```python
from build123d import *

# Parameters (mm, degrees)
SKETCH1_W           = 82.55
SKETCH1_H           = 69.85
BOSS_EXTRUDE1_DEPTH = 19.05
CUT_EXTRUDE2_START  = -19.05
SKETCH2_R           = 5.159375
CUT_EXTRUDE2_DEPTH  = 77.376117521
CUT_EXTRUDE4_START  = -19.05
SKETCH3_R           = 7.3421875
CUT_EXTRUDE4_DEPTH  = 28.575
CUT_EXTRUDE6_START  = -19.05
SKETCH4_R           = 12.7254
CUT_EXTRUDE6_DEPTH  = 2.8194
CUT_EXTRUDE8_START  = 41.275
SKETCH5_R           = 7.3421875
CUT_EXTRUDE8_DEPTH  = 60.325


with BuildPart() as part:
    # Sketch1 → Boss-Extrude1 (new, symmetric)
    with BuildSketch(Plane(origin=(0, 0, 0), x_dir=(1, 0, 0), z_dir=(0, 1, 0))):
        Rectangle(SKETCH1_W, SKETCH1_H)
    extrude(amount=BOSS_EXTRUDE1_DEPTH, both=True)

    # Sketch2 → Cut-Extrude2 (cut, through all)
    with BuildSketch(Plane(origin=(0, 0, 0), x_dir=(1, 0, 0), z_dir=(0, 1, 0)).offset(CUT_EXTRUDE2_START)):
        with Locations(Location((-30.1625, -23.8125, 0), (0, 0, 270))):
            Circle(SKETCH2_R)
        with Locations(Location((30.1625, -23.8125, 0), (0, 0, 270))):
            Circle(SKETCH2_R)
        with Locations(Location((-30.1625, 23.8125, 0), (0, 0, 270))):
            Circle(SKETCH2_R)
        with Locations(Location((30.1625, 23.8125, 0), (0, 0, 270))):
            Circle(SKETCH2_R)
    extrude(amount=CUT_EXTRUDE2_DEPTH, mode=Mode.SUBTRACT)

    # Sketch3 → Cut-Extrude4 (cut)
    with BuildSketch(Plane(origin=(0, 0, 0), x_dir=(1, 0, 0), z_dir=(0, 1, 0)).offset(CUT_EXTRUDE4_START)):
        with Locations(Location((-17.4625, 0, 0), (0, 0, 270))):
            Circle(SKETCH3_R)
        with Locations(Location((17.4625, 0, 0), (0, 0, 270))):
            Circle(SKETCH3_R)
    extrude(amount=CUT_EXTRUDE4_DEPTH, mode=Mode.SUBTRACT)

    # Sketch4 → Cut-Extrude6 (cut)
    with BuildSketch(Plane(origin=(0, 0, 0), x_dir=(1, 0, 0), z_dir=(0, 1, 0)).offset(CUT_EXTRUDE6_START)):
        with Locations(Location((-17.4625, 0, 0), (0, 0, 270))):
            Circle(SKETCH4_R)
        with Locations(Location((17.4625, 0, 0), (0, 0, 270))):
            Circle(SKETCH4_R)
    extrude(amount=CUT_EXTRUDE6_DEPTH, mode=Mode.SUBTRACT)

    # Sketch5 → Cut-Extrude8 (cut)
    with BuildSketch(Plane(origin=(0, 0, 0), x_dir=(0, 0, -1), z_dir=(1, 0, 0)).offset(CUT_EXTRUDE8_START)):
        Circle(SKETCH5_R)
    extrude(amount=-CUT_EXTRUDE8_DEPTH, mode=Mode.SUBTRACT)


solid = part.part
```
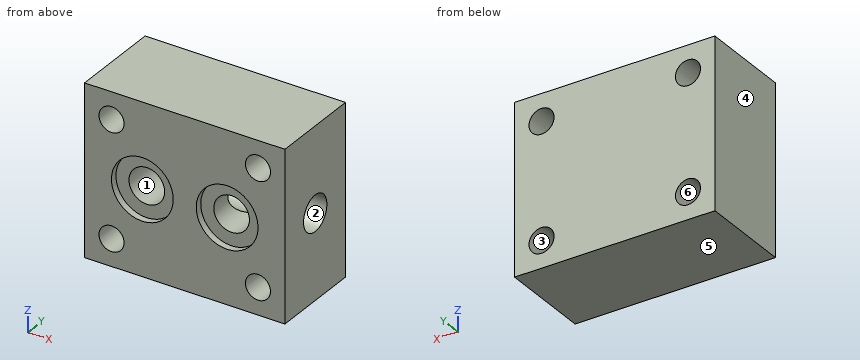
Check sheet for the modelled part. Datum: model origin and axes. Units: mm. Face numbers are marked on the shaded views. A direction names the side the tool comes from. Give positions to 0.01 mm unless a question says otherwise; leave off trailing zeros. Order: outer loops, then holes, each group sorted by start corner. A loop starts at its lowest first (then second) coordinate and runs counter-clockwise, first axis right, second up. Notation, with made-up numbers: (-14.75, 56.5) -> (32.25, 56.5) arc R18 ccw to (32.25, 64.5) -> close; hole circle Ø7 at (54, -31). An arc over 180 degrees is marked (long way). Use CSV: the item, a comma, the result in double quotes. Start each with the question number.
1) Mould release check, pull along Z, two halves, no side actions. Record for the marked faces 4, 5 and 6: released by +Z, released by -Z, zero draft, split by the parting line, or undercut.
2) Go/stop test with flat-tipped pins: P1, Ø4.5, axis at x = -20.5, z = 1.5, coming from the -Y side (3 decimals); P2, Ø16.5, axis at x = 30.16, z = 23.81, coming from the -Y side; P3, Ø17, axis at x = 17.46, z = 0, coming from the -Y side. Record where each tip stops, or that it passes through.
3) Sectioned sample at D-D, the plane z = -8.5. Record the boundary of the cut face in (x, y) (3 decimals).
4) Set-up check for the marked faces 1, 2 and 3: record each of +Z, -Z, +X, -X, +Y, -Y from which the full face is reachable in a straight line by a thin tool's end or side.
5) Sectioned sample at C-C, the plane y = 3. Record the boundary of the cut face in (x, z) (1 decimal).
6) Sectioned sample at B-B, the plane x = -1. Record the boundary of the cut face in (y, z) (3 decimals), plus the area to 3 significant figures.
7) Sectioned sample at A-A, the plane z = 0. Record the boundary of the cut face in (x, y) (3 decimals).
8) Material ranges on line 1 (X direction, y = -4, z = -24) (3 decimals); line 2 (X direction, y = -17, z = 0) (3 decimals); line 3 (Z direction, x = 32, y = 11) (3 decimals), recorded low to high. Write a range as from..to.
Recorded:
1,face 4,"zero draft"
1,face 5,"released by -Z"
1,face 6,"undercut"
2,P1,"y = 9.525"
2,P2,"y = -19.05"
2,P3,"y = -16.23"
3,outline,"(-41.275, -19.05) -> (-26.933, -19.05) -> (-26.933, -16.231) -> (-7.992, -16.231) -> (-7.992, -19.05) -> (7.992, -19.05) -> (7.992, -16.231) -> (26.933, -16.231) -> (26.933, -19.05) -> (41.275, -19.05) -> (41.275, 19.05) -> (-41.275, 19.05) -> close"
4,face 1,"-Y"
4,face 2,"+X"
4,face 3,"+Y, -Y"
5,outline,"(-41.3, -34.9) -> (41.3, -34.9) -> (41.3, -6.7) -> (20.5, -6.7) arc R7.3 cw to (14.5, -6.7) -> (-14.5, -6.7) arc R7.3 cw (long way) to (-14.5, 6.7) -> (14.5, 6.7) arc R7.3 cw to (20.5, 6.7) -> (41.3, 6.7) -> (41.3, 34.9) -> (-41.3, 34.9) -> close; hole circle Ø10.3 at (-30.2, -23.8); hole circle Ø10.3 at (-30.2, 23.8); hole circle Ø10.3 at (30.2, -23.8); hole circle Ø10.3 at (30.2, 23.8)"
6,outline,"(-19.05, -34.925) -> (19.05, -34.925) -> (19.05, 34.925) -> (-19.05, 34.925) -> close; hole circle Ø14.684 at (0, 0)"
6,area,"2,490 mm2"
7,outline,"(-41.275, -19.05) -> (-30.188, -19.05) -> (-30.188, -16.231) -> (-24.805, -16.231) -> (-24.805, 9.525) -> (-10.12, 9.525) -> (-10.12, 7.342) -> (10.12, 7.342) -> (10.12, 9.525) -> (24.805, 9.525) -> (24.805, 7.342) -> (41.275, 7.342) -> (41.275, 19.05) -> (-41.275, 19.05) -> close; (-10.12, -16.231) -> (-4.737, -16.231) -> (-4.737, -19.05) -> (4.737, -19.05) -> (4.737, -16.231) -> (10.12, -16.231) -> (10.12, -7.342) -> (-10.12, -7.342) -> close; (24.805, -16.231) -> (30.188, -16.231) -> (30.188, -19.05) -> (41.275, -19.05) -> (41.275, -7.342) -> (24.805, -7.342) -> close"
8,line 1,"-41.275..-35.318, -25.007..25.007, 35.318..41.275"
8,line 2,"-41.275..-30.188, -4.737..4.737, 30.188..41.275"
8,line 3,"-34.925..-28.634, -18.991..18.991, 28.634..34.925"
